For this review, take the finished solid that the model builds, in its own axes (mm). Face numbers are marked on the shaded views. A direction names the side the tool comes from. Coordinates: 2 decimals unless noted, no trailing zeros. Write each loop counter-clockwise with the first axis right and the second up, starting at its lowest first coordinate (ties: lowest second). Pieces come first, ordered by that corner, then holes. Notation, with made-up numbers: M 41,-16.5 L 91,-16.5 A23 ccw 91,12.5 Z; hole C -19,75 d3. An arc over 180 degrees is marked long. One line per question, with ' | ' between items.
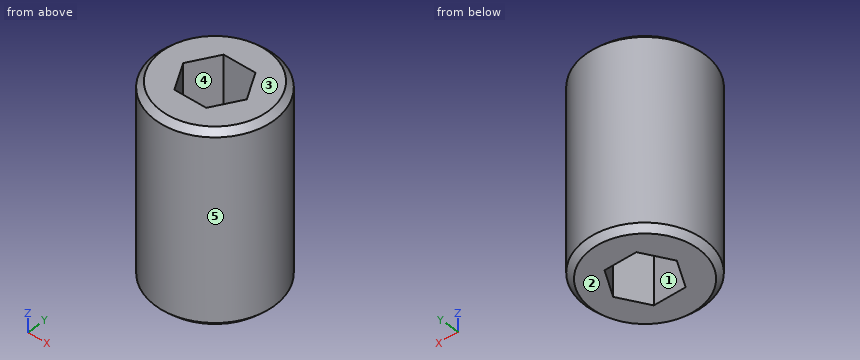
from build123d import *

# Parameters (mm, degrees)
SKETCH1_R           = 10.16
BOSS_EXTRUDE1_DEPTH = 33.02
CHAMFER1_SIZE       = 1


with BuildPart() as part:
    # Sketch1 → Boss-Extrude1 (new body)
    with BuildSketch(Plane.XY):
        Circle(SKETCH1_R)
        Polygon((5.499261314, 0), (2.749630657, 4.7625), (-2.749630657, 4.7625), (-5.499261314, 0), (-2.749630657, -4.7625), (2.749630657, -4.7625), align=None, mode=Mode.SUBTRACT)
    extrude(amount=BOSS_EXTRUDE1_DEPTH)

    # Chamfer1
    chamfer1_edges = [part.edges().sort_by_distance(p)[0] for p in [
        (-10.16, 0, 0),
        (-10.16, 0, 33.02),
    ]]
    chamfer(chamfer1_edges, length=CHAMFER1_SIZE)


solid = part.part
1) We need section A-A on x = 0. State the section outline as (y, z) points.
Responses:
outline: M -10.16,1 L -9.16,0 L -4.76,0 L -4.76,33.02 L -9.16,33.02 L -10.16,32.02 Z; M 4.76,0 L 9.16,0 L 10.16,1 L 10.16,32.02 L 9.16,33.02 L 4.76,33.02 Z
2) Insertion check: pin 1 Ø2 at (x, z) = (6, 15) entering from -Y; pin 2 Ø4 at (y, z) = (-5.5, 6.5) entering from -X; pin 3 Ø1.6 at (x, z) = (-1, 10.5) entering from +Y; pin 4 Ø10 at (x, y) = (5.5, -2) entering from -Z. Each pin has a flat end and moves straight along its axis. Give the tip position at first contact, or say it passes through.
Responses:
pin 1: y = -8.84 | pin 2: x = -9.54 | pin 3: y = 10.16 | pin 4: z = 0
3) Machinability: for the marked faces 1 and 2, which of the approach directions +Z, -Z, +X, -X, +Y, -Y give a long, thin tool a straight path to every point of the face, cutting with its end or side? Answer none if there is none.
Responses:
face 1: +Z, -Z | face 2: -Z, +X, -X, +Y, -Y
4) The part is to be moulded in two halves that separate along Y. For the marked faces 3, 4 and 5, say which applies: +Y half, -Y half, draft (parallel to the pull), parting line (faces both ways), or undercut.
Responses:
face 3: draft | face 4: undercut | face 5: parting line
5) We need section B-B on z = 13.5. State the section outline as (x, y) points.
Responses:
outline: C 0,0 d20.32; hole M -5.5,0 L -2.75,-4.76 L 2.75,-4.76 L 5.5,0 L 2.75,4.76 L -2.75,4.76 Z
6) To check wall thickness, follow line 1 along Y through (x, z) = (0.25, 22); line 2 along X through (y, z) = (-1.75, 7); line 3 along X through (y, z) = (3, 24). State the ranges of each line that lie inside material, in increasing order. Write a range as [from, to].
Responses:
line 1: [-10.16, -4.76], [4.76, 10.16] | line 2: [-10.01, -4.49], [4.49, 10.01] | line 3: [-9.71, -3.77], [3.77, 9.71]
